Build history of the part. All positions in model axes, mm. Round coordinates to 2 decimals unless told otherwise and drop trailing zeros. Write each loop counter-clockwise with the first axis right and the second up, starting at its lowest first coordinate (ties: lowest second). Pieces come first, ordered by that corner, then holes.
from build123d import *

# Parameters (mm, degrees)
SKETCH1_R               = 17.78
BOSS_EXTRUDE1_DEPTH     = 50.8
SKETCH2_R               = 16.764
CUT_EXTRUDE1_DEPTH      = 177.8
CUT_EXTRUDE3_DEPTH      = 8.128
CUT_EXTRUDE5_DEPTH      = 8.128
CUT_EXTRUDE6_DEPTH      = 57.682420555
CUT_EXTRUDE6_DEPTH_BACK = 57.682420555
SKETCH8_W               = 2.16473232
SKETCH8_H               = 8.128


with BuildPart() as part:
    # Sketch1 → Boss-Extrude1 (new body)
    with BuildSketch(Plane(origin=(0, 0, 0), x_dir=(1, 0, 0), z_dir=(0, 1, 0))):
        with Locations(Location((0, 0, 0), (0, 0, 270))):
            Circle(SKETCH1_R)
    extrude(amount=BOSS_EXTRUDE1_DEPTH)

    # Sketch2 → Cut-Extrude1 (cut)
    with BuildSketch(Plane(origin=(0, 50.8, 0), x_dir=(1, 0, 0), z_dir=(0, 1, 0))):
        with Locations(Location((0, 0, 0), (0, 0, 270))):
            Circle(SKETCH2_R)
    extrude(amount=-CUT_EXTRUDE1_DEPTH, mode=Mode.SUBTRACT)

    # Sketch5 → Cut-Extrude3 (cut)
    with BuildSketch(Plane(origin=(0, 0, 0), x_dir=(1, 0, 0), z_dir=(0, 1, 0))):
        with BuildLine():
            Line((17.78, 2.54), (-17.78, 2.54))
            ThreePointArc((-17.78, 2.54), (0, 20.32), (17.78, 2.54))
        make_face()
    extrude(amount=CUT_EXTRUDE3_DEPTH, mode=Mode.SUBTRACT)

    # Sketch6 → Cut-Extrude5 (cut)
    with BuildSketch(Plane(origin=(0, 0, 0), x_dir=(1, 0, 0), z_dir=(0, 1, 0))):
        with BuildLine():
            Line((17.78, -2.54), (-17.78, -2.54))
            ThreePointArc((-17.78, -2.54), (0, -18.882130931), (17.78, -2.54))
        make_face()
    extrude(amount=CUT_EXTRUDE5_DEPTH, mode=Mode.SUBTRACT)

    # Sketch8 → Cut-Extrude6 (cut, two sides: drawn at the far end of the back side and taken through both)
    with BuildSketch(Plane.XY.offset(-CUT_EXTRUDE6_DEPTH_BACK)):
        with Locations((17.267156574, 4.064)):
            Rectangle(SKETCH8_W, SKETCH8_H)
    extrude(amount=CUT_EXTRUDE6_DEPTH + CUT_EXTRUDE6_DEPTH_BACK, mode=Mode.SUBTRACT)


solid = part.part
1) Wall check: L1, parallel to X at y = 11, z = 0; L2, parallel to Y at x = 10, z = 14. Give the ranges that are in metal, low to high.
Results:
L1: x = -17.78 to -16.76, 16.76 to 17.78
L2: y = 8.13 to 50.8
2) Slice it at A-A (z = 0). Write the cut outline in (x, y), plus the area to 3 significant figures.
Results:
outline: (-17.78, 0) - (-16.76, 0) - (-16.76, 50.8) - (-17.78, 50.8) - close; (16.76, 8.13) - (17.78, 8.13) - (17.78, 50.8) - (16.76, 50.8) - close
area: 95.0 mm2
3) Slice it at D-D (y = 6). Write the cut outline in (x, z), plus the area to 3 significant figures.
Results:
outline: (-17.6, -2.54) - (-16.57, -2.54) arc R16.76 cw to (-16.57, 2.54) - (-17.6, 2.54) arc R17.78 ccw to start
area: 5.18 mm2
4) Slice it at C-C (y = 42). Write the cut outline in (x, z).
Results:
outline: circle Ø35.56 at (0, 0); hole circle Ø33.53 at (0, 0)
5) Slice it at B-B (x = 0). Write the cut outline in (y, z), plus the area to 3 significant figures.
Results:
outline: (8.13, -17.78) - (50.8, -17.78) - (50.8, -16.76) - (8.13, -16.76) - close; (8.13, 16.76) - (50.8, 16.76) - (50.8, 17.78) - (8.13, 17.78) - close
area: 86.7 mm2
6) Pin check, flat tips, straight feed: pin 1 Ø3 at (y, z) = (10, 7.5) entering from +X; pin 2 Ø20 at (x, z) = (0, 0) entering from -Y; pin 3 Ø0.5 at (x, y) = (-17.5, 3.5) entering from +Z; pin 4 Ø5 at (y, z) = (34.5, 11.5) entering from +X. Stop position of each tip, or through.
Results:
pin 1: stops at x = 16.74
pin 2: passes through
pin 3: stops at z = 2.54
pin 4: stops at x = 15.33
7) Mould opens along X. For faces 1 (the cylindrical face through (-14.87, 25.76, 7.74)), 2 (the flat face through (12, 50.8, -12)), 3 (the cylindrical face through (-15.774, 30.689, 8.204)) say: released by +X, released by -X, zero draft, split by the parting line, or undercut.
Results:
face 1: undercut
face 2: zero draft
face 3: split by the parting line
